```python
from build123d import *

# Parameters (mm, degrees)
F0_W           = 25
F0_H           = 12
F0_W_2         = 19
F0_H_2         = 8
F1_DEPTH       = 10
F2_W           = 21
F2_H           = 8
F2_W_2         = 17
F2_H_2         = 2
F3_DEPTH       = 25
F4_W           = 21
F4_H           = 8
F4_W_2         = 17
F4_H_2         = 2
F5_DEPTH       = 2
F6_W           = 25
F6_H           = 12
F7_DEPTH       = 4
F10_DEPTH      = 4
F10_DEPTH_BACK = 4
F11_T1_DEPTH   = 21
F11_T3_DEPTH   = 8
F11_T9_DEPTH   = 31
F11_T14_DEPTH  = 18
F11_T22_DEPTH  = 31
F11_T27_DEPTH  = 18
F11_T35_DEPTH  = 31
F11_T40_DEPTH  = 18
F11_T48_DEPTH  = 18
F11_T53_DEPTH  = 31
F12_R          = 1
F14_DEPTH      = 1


# Not quite as in the source:
# - a fillet or chamfer that OpenCascade refuses, or shapes differently, is made with other operations: its cross-section is extruded or revolved along the edge and cut away or added


with BuildPart() as f1:
    # F0 (on Top) → F1 (new body)
    with BuildSketch(Plane.XY):
        with Locations((12.5, 6)):
            Rectangle(F0_W, F0_H)
        with Locations((12.5, 6)):
            Rectangle(F0_W_2, F0_H_2, mode=Mode.SUBTRACT)
    extrude(amount=-F1_DEPTH)

    # F2 (on Top) → F3 (join)
    with BuildSketch(Plane.XY):
        with Locations((12.5, 6)):
            Rectangle(F2_W, F2_H)
        with Locations((12.5, 6)):
            Rectangle(F2_W_2, F2_H_2, mode=Mode.SUBTRACT)
    extrude(amount=F3_DEPTH)

    # F4 (on face) → F5 (join)
    with BuildSketch(Plane.XY.offset(25)):
        with Locations((12.5, 6)):
            Rectangle(F4_W, F4_H)
        with Locations((12.5, 6)):
            Rectangle(F4_W_2, F4_H_2, mode=Mode.SUBTRACT)
        with Locations((12.5, 6)):
            Rectangle(F4_W_2, F4_H_2)
    extrude(amount=F5_DEPTH)

    # F6 (on face) → F7 (join)
    with BuildSketch(Plane.XY):
        with Locations((12.5, 6)):
            Rectangle(F6_W, F6_H)
        Polygon((23, 2), (22, 2), (3, 2), (2, 2), (2, 10), (3, 10), (22, 10), (23, 10), align=None, mode=Mode.SUBTRACT)
    extrude(amount=F7_DEPTH)

    # F9 (on offset) → F10 (join, two sides)
    with BuildSketch(Plane.XZ.offset(-6)) as f10_sk:
        with BuildLine():
            Line((3, -7), (3, -8.5))
            Line((3, -8.5), (3.4671572875, -8.0328427125))
            ThreePointArc((3.4671572875, -8.0328427125), (3.5843145751, -7.75), (3.4671572875, -7.4671572875))
            Line((3.4671572875, -7.4671572875), (3, -7))
        make_face()
        with BuildLine():
            Line((21.5328427125, -8.0328427125), (22, -8.5))
            Line((22, -8.5), (22, -7))
            Line((22, -7), (21.5328427125, -7.4671572875))
            ThreePointArc((21.5328427125, -7.4671572875), (21.4156854249, -7.75), (21.5328427125, -8.0328427125))
        make_face()
    extrude(amount=F10_DEPTH)
    extrude(f10_sk.sketch, amount=-F10_DEPTH_BACK)

    # F11: fillet of radius 5 on 4 edges, made by hand

    # F11_s2 → F11_t1 (join)
    with BuildSketch(Plane.YZ.offset(2)):
        with BuildLine():
            ThreePointArc((0, 4), (1.472135955, 5.7639320225), (2, 8))
            Line((2, 8), (2, 4))
            Line((2, 4), (0, 4))
        make_face()
        with BuildLine():
            ThreePointArc((12, 4), (10.527864045, 5.7639320225), (10, 8))
            Line((10, 8), (10, 4))
            Line((10, 4), (12, 4))
        make_face()
    extrude(amount=F11_T1_DEPTH)

    # F11_s4 → F11_t3 (join)
    with BuildSketch(Plane.XZ.offset(-10)):
        with BuildLine():
            ThreePointArc((25, 4), (23.527864045, 5.7639320225), (23, 8))
            Line((23, 8), (23, 4))
            Line((23, 4), (25, 4))
        make_face()
        with BuildLine():
            ThreePointArc((0, 4), (1.472135955, 5.7639320225), (2, 8))
            Line((2, 8), (2, 4))
            Line((2, 4), (0, 4))
        make_face()
    extrude(amount=F11_T3_DEPTH)


with BuildPart() as f11_tool7:
    # F11_s8 → F11_t9 (new body)
    with BuildSketch(Plane.YZ.offset(-8)):
        with BuildLine():
            ThreePointArc((0, 4), (1.472135955, 5.7639320225), (2, 8))
            Line((2, 8), (2, 4))
            Line((2, 4), (0, 4))
        make_face()
    extrude(amount=F11_T9_DEPTH)

    split(bisect_by=Plane.YZ, keep=Keep.TOP)

    split(bisect_by=Plane.YZ.offset(2), keep=Keep.BOTTOM)


with BuildPart() as f11_tool12:
    # F11_s13 → F11_t14 (new body)
    with BuildSketch(Plane.XZ.offset(8)):
        with BuildLine():
            ThreePointArc((0, 4), (1.472135955, 5.7639320225), (2, 8))
            Line((2, 8), (2, 4))
            Line((2, 4), (0, 4))
        make_face()
    extrude(amount=-F11_T14_DEPTH)

    split(bisect_by=Plane.XZ, keep=Keep.BOTTOM)

    split(bisect_by=Plane.XZ.offset(-2), keep=Keep.TOP)


with BuildPart() as f11_tool7_1:
    add(f11_tool7.part)

    # F11_t17: intersect F11_tool12
    add(f11_tool12.part, mode=Mode.INTERSECT)


with BuildPart() as f1_1:
    add(f1.part)

    # F11_t5: union F11_tool7
    add(f11_tool7_1.part)


with BuildPart() as f11_tool20:
    # F11_s21 → F11_t22 (new body)
    with BuildSketch(Plane.YZ.offset(2)):
        with BuildLine():
            ThreePointArc((0, 4), (1.472135955, 5.7639320225), (2, 8))
            Line((2, 8), (2, 4))
            Line((2, 4), (0, 4))
        make_face()
    extrude(amount=F11_T22_DEPTH)

    split(bisect_by=Plane.YZ.offset(25), keep=Keep.BOTTOM)

    split(bisect_by=Plane.YZ.offset(23), keep=Keep.TOP)


with BuildPart() as f11_tool25:
    # F11_s26 → F11_t27 (new body)
    with BuildSketch(Plane.XZ.offset(-10)):
        with BuildLine():
            ThreePointArc((25, 4), (23.527864045, 5.7639320225), (23, 8))
            Line((23, 8), (23, 4))
            Line((23, 4), (25, 4))
        make_face()
    extrude(amount=F11_T27_DEPTH)

    split(bisect_by=Plane.XZ, keep=Keep.BOTTOM)

    split(bisect_by=Plane.XZ.offset(-2), keep=Keep.TOP)


with BuildPart() as f11_tool20_1:
    add(f11_tool20.part)

    # F11_t30: intersect F11_tool25
    add(f11_tool25.part, mode=Mode.INTERSECT)


with BuildPart() as f1_2:
    add(f1_1.part)

    # F11_t18: union F11_tool20
    add(f11_tool20_1.part)


with BuildPart() as f11_tool33:
    # F11_s34 → F11_t35 (new body)
    with BuildSketch(Plane.YZ.offset(33)):
        with BuildLine():
            ThreePointArc((12, 4), (10.527864045, 5.7639320225), (10, 8))
            Line((10, 8), (10, 4))
            Line((10, 4), (12, 4))
        make_face()
    extrude(amount=-F11_T35_DEPTH)

    split(bisect_by=Plane.YZ.offset(25), keep=Keep.BOTTOM)

    split(bisect_by=Plane.YZ.offset(23), keep=Keep.TOP)


with BuildPart() as f11_tool38:
    # F11_s39 → F11_t40 (new body)
    with BuildSketch(Plane.XZ.offset(-20)):
        with BuildLine():
            ThreePointArc((25, 4), (23.527864045, 5.7639320225), (23, 8))
            Line((23, 8), (23, 4))
            Line((23, 4), (25, 4))
        make_face()
    extrude(amount=F11_T40_DEPTH)

    split(bisect_by=Plane.XZ.offset(-12), keep=Keep.TOP)

    split(bisect_by=Plane.XZ.offset(-10), keep=Keep.BOTTOM)


with BuildPart() as f11_tool33_1:
    add(f11_tool33.part)

    # F11_t43: intersect F11_tool38
    add(f11_tool38.part, mode=Mode.INTERSECT)


with BuildPart() as f1_3:
    add(f1_2.part)

    # F11_t31: union F11_tool33
    add(f11_tool33_1.part)


with BuildPart() as f11_tool46:
    # F11_s47 → F11_t48 (new body)
    with BuildSketch(Plane.XZ.offset(-2)):
        with BuildLine():
            ThreePointArc((0, 4), (1.472135955, 5.7639320225), (2, 8))
            Line((2, 8), (2, 4))
            Line((2, 4), (0, 4))
        make_face()
    extrude(amount=-F11_T48_DEPTH)

    split(bisect_by=Plane.XZ.offset(-12), keep=Keep.TOP)

    split(bisect_by=Plane.XZ.offset(-10), keep=Keep.BOTTOM)


with BuildPart() as f11_tool51:
    # F11_s52 → F11_t53 (new body)
    with BuildSketch(Plane.YZ.offset(23)):
        with BuildLine():
            ThreePointArc((12, 4), (10.527864045, 5.7639320225), (10, 8))
            Line((10, 8), (10, 4))
            Line((10, 4), (12, 4))
        make_face()
    extrude(amount=-F11_T53_DEPTH)

    split(bisect_by=Plane.YZ, keep=Keep.TOP)

    split(bisect_by=Plane.YZ.offset(2), keep=Keep.BOTTOM)


with BuildPart() as f11_tool46_1:
    add(f11_tool46.part)

    # F11_t56: intersect F11_tool51
    add(f11_tool51.part, mode=Mode.INTERSECT)


with BuildPart() as f1_4:
    add(f1_3.part)

    # F11_t44: union F11_tool46
    add(f11_tool46_1.part)

    # F12
    f12_edges = [f1_4.edges().sort_by_distance(p)[0] for p in [
        (23, 6, 27),
        (12.5, 2, 27),
        (2, 6, 27),
        (12.5, 10, 27),
        (12.5, 12, 4),
        (25, 6, 4),
        (12.5, 0, 4),
        (0, 6, 4),
    ]]
    fillet(f12_edges, radius=F12_R)

    # F13 (on face) → F14 (cut)
    with BuildSketch(Plane(origin=(0, 10, 0), x_dir=(-1, 0, 0), z_dir=(0, 1, 0))):
        Polygon((-12.5, 20.9), (-17, 13.1057713659), (-8, 13.1057713659), align=None)
        with BuildLine():
            Line((-12.75, 13.6057713659), (-16.1339745962, 13.6057713659))
            Line((-16.1339745962, 13.6057713659), (-14.4419872981, 16.536379332))
            Line((-14.4419872981, 16.536379332), (-14.4290420842, 16.5289054093))
            ThreePointArc((-14.4290420842, 16.5289054093), (-14.3169872981, 14.6548094716), (-12.75, 13.6207192114))
            Line((-12.75, 13.6207192114), (-12.75, 13.6057713659))
        make_face(mode=Mode.SUBTRACT)
        with BuildLine():
            ThreePointArc((-12.75, 14.125447255), (-14.0980762114, 15.7038475773), (-12.75, 17.2822478995))
            Line((-12.75, 17.2822478995), (-12.75, 14.125447255))
        make_face(mode=Mode.SUBTRACT)
        with BuildLine():
            ThreePointArc((-12.25, 17.2822478995), (-10.9019237886, 15.7038475773), (-12.25, 14.125447255))
            Line((-12.25, 14.125447255), (-12.25, 17.2822478995))
        make_face(mode=Mode.SUBTRACT)
        with BuildLine():
            Line((-8.8660254038, 13.6057713659), (-12.25, 13.6057713659))
            Line((-12.25, 13.6057713659), (-12.25, 13.6207192114))
            ThreePointArc((-12.25, 13.6207192114), (-10.6830127019, 14.6548094716), (-10.5709579158, 16.5289054093))
            Line((-10.5709579158, 16.5289054093), (-10.5580127019, 16.536379332))
            Line((-10.5580127019, 16.536379332), (-8.8660254038, 13.6057713659))
        make_face(mode=Mode.SUBTRACT)
        with BuildLine():
            Line((-12.75, 19.4669872981), (-12.75, 17.7869759432))
            ThreePointArc((-12.75, 17.7869759432), (-13.5490381057, 17.5208348754), (-14.1790420842, 16.9619181112))
            Line((-14.1790420842, 16.9619181112), (-14.1919872981, 16.9693920339))
            Line((-14.1919872981, 16.9693920339), (-12.75, 19.4669872981))
        make_face(mode=Mode.SUBTRACT)
        with BuildLine():
            Line((-12.25, 17.7869759432), (-12.25, 19.4669872981))
            Line((-12.25, 19.4669872981), (-10.8080127019, 16.9693920339))
            Line((-10.8080127019, 16.9693920339), (-10.8209579158, 16.9619181112))
            ThreePointArc((-10.8209579158, 16.9619181112), (-11.4509618943, 17.5208348754), (-12.25, 17.7869759432))
        make_face(mode=Mode.SUBTRACT)
    extrude(amount=-F14_DEPTH, mode=Mode.SUBTRACT)


solid = f1_4.part
```
Work out the finished part from the listing and answer in its coordinate system (mm). A direction names the side the tool comes from. Round coordinates to 2 decimals unless told otherwise and drop trailing zeros. Order: outer loops, then holes, each group sorted by start corner. A loop starts at its lowest first (then second) coordinate and runs counter-clockwise, first axis right, second up.
Q1. The mould has two halves that part along X. Classify faces 1 (the cylindrical face through (22.715, 6.056, 26.699)), 2 (the flat face through (13.48, 9.51, 18.2)), 3 (the flat face through (10, 10, 17)): pulls with the +X half, pulls with the -X half, needs draft (parallel to the pull), parting line crosses it, or undercut.
Solution:
face 1: pulls with the +X half
face 2: undercut
face 3: needs draft
Q2. Given pin 1 Ø0.6 at (y, z) = (6.5, 10.5) entering from -X; pin 2 Ø4 at (x, y) = (10.5, 5) entering from -Z; pin 3 Ø1.2 at (x, z) = (11.5, 18) entering from +Y, each flat-ended and moving along its own axis, determine where each tip first touches the part or whether it passes through.
Solution:
pin 1: stops at x = 2
pin 2: stops at z = 0
pin 3: stops at y = 10
Q3. A tool of negligible diameter and unlimited length cuts with its end or side. For faces 4 (the flat face through (12, 12, -3)), 5 (the flat face through (12, 7, 12)), 6 (the flat face through (13, 10, 18)), 7 (the flat face through (22, 6, -3)), 8 (the flat face through (12.25, 9.5, 18.6)), from which of +Z, -Z, +X, -X, +Y, -Y can it reach the whole face along a straight path? Write none if from no direction.
Solution:
face 4: +Z, -Z, +X, -X, +Y
face 5: -Z
face 6: +Z, +X, -X, +Y
face 7: none
face 8: +Y
Q4. A cutting plane is placed at A-A, the plane z = 11.5. Determine the outline of the cut face in (x, y).
Solution:
outline: (2, 2) - (23, 2) - (23, 10) - (2, 10) - close; hole (4, 5) - (21, 5) - (21, 7) - (4, 7) - close
Q5. Find the intervals of material crossed by line 1 along Y through (x, z) = (4.75, -7); line 2 along Y through (x, z) = (13.25, 2); line 3 along X through (y, z) = (8.25, -3.5), in increasing order.
Solution:
line 1: y = 0 to 2, 10 to 12
line 2: y = 0 to 5, 7 to 12
line 3: x = 0 to 3, 22 to 25
Q6. A cutting plane is placed at D-D, the plane z = -2.5. Determine the outline of the cut face in (x, y).
Solution:
outline: (0, 0) - (25, 0) - (25, 12) - (0, 12) - close; hole (3, 2) - (22, 2) - (22, 10) - (3, 10) - close
Q7. A cutting plane is placed at B-B, the plane x = 20.5. Determine the outline of the cut face in (y, z).
Solution:
outline: (0, -10) - (2, -10) - (2, 0) - (5, 0) - (5, 25) - (7, 25) - (7, 0) - (10, 0) - (10, -10) - (12, -10) - (12, 3.53) arc R1 ccw to (11.67, 4.27) arc R5 cw to (10, 8) - (10, 26) arc R1 ccw to (9, 27) - (3, 27) arc R1 ccw to (2, 26) - (2, 8) arc R5 cw to (0.33, 4.27) arc R1 ccw to (0, 3.53) - close
Q8. A cutting plane is placed at C-C, the plane y = 7.5. Determine the outline of the cut face in (x, z), then the cut area to 3 significant figures.
Solution:
outline: (0, -10) - (3, -10) - (3, -8.5) - (3.47, -8.03) arc R0.4 ccw to (3.47, -7.47) - (3, -7) - (3, 0) - (22, 0) - (22, -7) - (21.53, -7.47) arc R0.4 ccw to (21.53, -8.03) - (22, -8.5) - (22, -10) - (25, -10) - (25, 3.53) arc R1 ccw to (24.67, 4.27) arc R5 cw to (23, 8) - (23, 26) arc R1 ccw to (22, 27) - (3, 27) arc R1 ccw to (2, 26) - (2, 8) arc R5 cw to (0.33, 4.27) arc R1 ccw to (0, 3.53) - close
area: 648 mm2
